from build123d import *

# Parameters (mm, degrees)
PAD001_DEPTH = 2
PAD_DEPTH    = 2


with BuildPart() as star:
    # Sketch001 → Pad001 (new body)
    with BuildSketch(Plane.XY):
        Polygon((0, 112.610254), (2.5, 108.280127), (7.5, 108.280127), (5, 103.95), (7.5, 99.619873), (2.5, 99.619873), (0, 95.289746), (-2.5, 99.619873), (-7.5, 99.619873), (-5, 103.95), (-7.5, 108.280127), (-2.5, 108.280127), align=None)
    extrude(amount=PAD001_DEPTH)


with BuildPart() as fusion:
    # Sketch → Pad (new body)
    with BuildSketch(Plane.XY):
        with BuildLine():
            Line((7.5, 0), (-7.5, 0))
            Line((-7.5, 0), (-7.5, 15))
            ThreePointArc((-41.967689, 15), (-24.733845, 11.812809), (-7.5, 15))
            Line((0, 105), (-41.967689, 15))
            Line((0, 105), (41.967689, 15))
            ThreePointArc((7.5, 15), (24.733845, 11.812809), (41.967689, 15))
            Line((7.5, 15), (7.5, 0))
        make_face()
    extrude(amount=PAD_DEPTH)

    # Fusion: union Star
    add(star.part)


solid = fusion.part
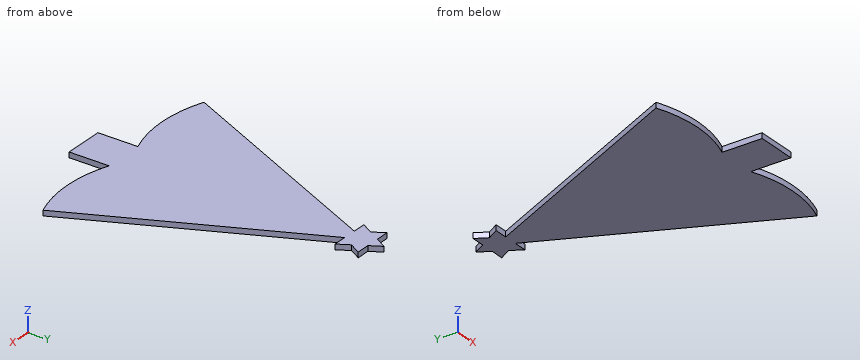
Geometry check sheet. Reference: the model listing, model coordinates, mm. Round coordinates to 2 decimals unless told otherwise and drop trailing zeros. Order: outer loops, then holes, each group sorted by start corner. A loop starts at its lowest first (then second) coordinate and runs counter-clockwise, first axis right, second up. Notation, with made-up numbers: (80, -27.5) - (134, -27.5) arc R21 ccw to (134, -0.5) - close; hole circle Ø7 at (-5, 40.25). An arc over 180 degrees is marked (long way). One line per question, with ' | ' between items. Start each with the question number.
(1) Sectioned sample at A-A on z = 1.1. Record the cut outline in (x, y).
(2) Depth check by flat-ended pin: pin 1 Ø1 at (x, z) = (-4, 1.5) entering from +Y; pin 2 Ø1 at (y, z) = (49.5, 1.5) entering from +X; pin 3 Ø0.6 at (y, z) = (6.5, 0.5) entering from -X. Enter the tip coordinate at first touch or a pass-through.
(3) Sectioned sample at B-B on x = 25. Record the cut outline in (y, z), and give its area (3 significant figures).
(4) Thickness scan on L1, parallel to X at y = 97, z = 1.7; L2, parallel to X at y = 5, z = 0.45; L3, parallel to Y at x = 32, z = 0.6. Record the ranges inside material, lowest first. Write a range as [from, to].
(5) Sectioned sample at C-C on y = 69. Record the cut outline in (x, z), and give its area (3 significant figures).
Conclusion:
1) outline: (-41.97, 15) arc R48.19 ccw to (-7.5, 15) - (-7.5, 0) - (7.5, 0) - (7.5, 15) arc R48.19 ccw to (41.97, 15) - (2.51, 99.62) - (7.5, 99.62) - (5, 103.95) - (7.5, 108.28) - (2.5, 108.28) - (0, 112.61) - (-2.5, 108.28) - (-7.5, 108.28) - (-5, 103.95) - (-7.5, 99.62) - (-2.51, 99.62) - close
2) pin 1: stops at y = 108.28 | pin 2: stops at x = 26.11 | pin 3: stops at x = -7.5
3) outline: (11.81, 0) - (51.39, 0) - (51.39, 2) - (11.81, 2) - close | area: 79.1 mm2
4) L1: x = [-3.73, 3.73] | L2: x = [-7.5, 7.5] | L3: y = [12.36, 36.38]
5) outline: (-16.79, 0) - (16.79, 0) - (16.79, 2) - (-16.79, 2) - close | area: 67.1 mm2
